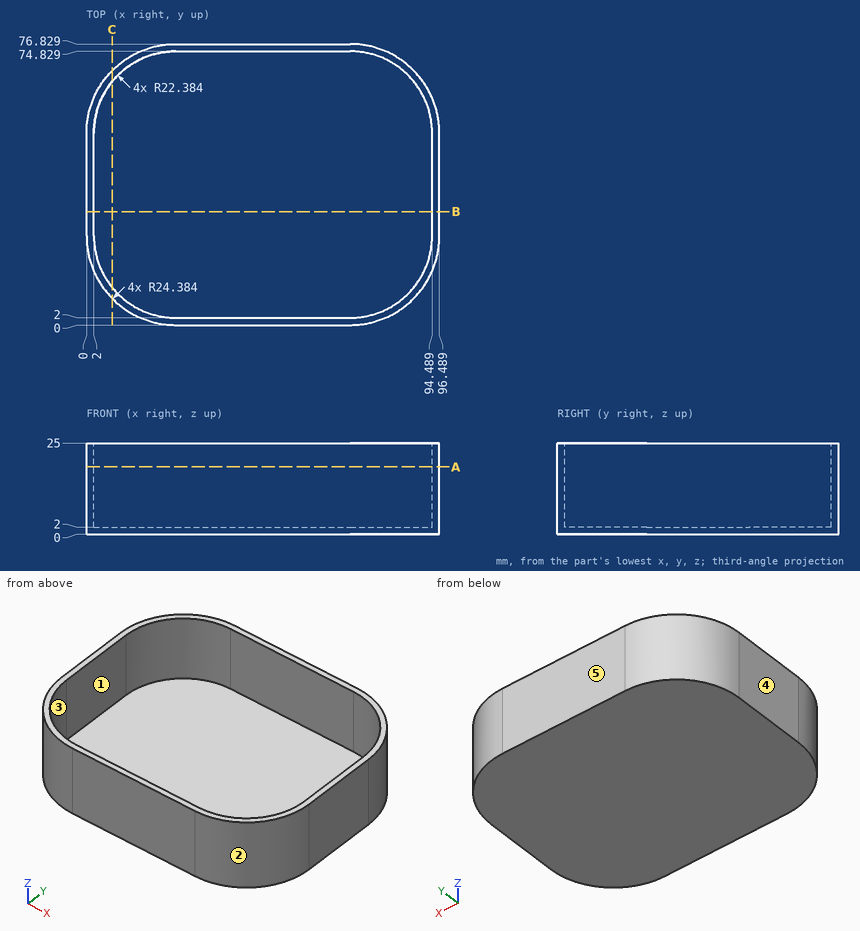
Print and shaded views of the part. All mm, measured from the part's lowest x, y and z. A direction names the side the tool comes from. Coordinates: 2 decimals unless noted, no trailing zeros. Loops run counter-clockwise (first coordinate to the right, second up) from the corner with the lowest first, then second, coordinate; pieces in that order, holes last. Notation, with made-up numbers: (59, 31.5) -> (112, 31.5) arc R35 ccw to (112, 70.5) -> close; hole circle Ø1 at (35, 60). An arc over 180 degrees is marked (long way). Use one line per item in the form item = value. Start each with the question number.
(1) Cut at A-A on z = 18.5. Give the cut face in (x, y) (1 decimal).
(2) Pull direction Y, two halves, no side cores. Call the marked faces 3, 4 and 5: pulls with the +Y half, pulls with the -Y half, needs draft (parallel to the pull), parting line crosses it, or undercut.
(3) Cut at B-B on y = 31. Give the cut face in (x, z), and give its area (3 significant figures).
(4) Cut at C-C on x = 7. Give the cut face in (y, z) (1 decimal).
(5) Tool access for the marked faces 1 and 2: list every direction of +Z, -Z, +X, -X, +Y, -Y with a clear straight run to the whole face (end or side of a thin tool).
(6) Flat gauge pins, fed straight in: pin 1 (8 mm diameter, centred on x = 85.5, z = 17.5, fed in from +Y); pin 2 (6 mm diameter, centred on y = 9, z = 5.5, fed in from -X); pin 3 (12 mm diameter, centred on x = 39, y = 30, fed in from +Z). Where does each tip first touch, or does it go through?
(7) Probe probe 1 along Y at (x, z) = (24, 21.5) (1 decimal); probe 2 along X at (y, z) = (45.5, 8); probe 3 along Z at (x, y) = (76, 57). List the from-to ranges inside material, lowest first. Write a range as from..to.
Values:
q1.outline = (0, 24.4) arc R24.4 ccw to (24.4, 0) -> (72.1, 0) arc R24.4 ccw to (96.5, 24.4) -> (96.5, 52.4) arc R24.4 ccw to (72.1, 76.8) -> (24.4, 76.8) arc R24.4 ccw to (0, 52.4) -> close; hole (2, 24.4) arc R22.4 ccw to (24.4, 2) -> (72.1, 2) arc R22.4 ccw to (94.5, 24.4) -> (94.5, 52.4) arc R22.4 ccw to (72.1, 74.8) -> (24.4, 74.8) arc R22.4 ccw to (2, 52.4) -> close
q2.face_3 = undercut
q2.face_4 = needs draft
q2.face_5 = pulls with the +Y half
q3.outline = (0, 0) -> (96.49, 0) -> (96.49, 25) -> (94.49, 25) -> (94.49, 2) -> (2, 2) -> (2, 25) -> (0, 25) -> close
q3.area = 285 mm2
q4.outline = (7.3, 0) -> (69.5, 0) -> (69.5, 25) -> (66.5, 25) -> (66.5, 2) -> (10.3, 2) -> (10.3, 25) -> (7.3, 25) -> close
q5.face_1 = +Z
q5.face_2 = +Z, -Z, +X, -Y
q6.pin_1 = 74.95
q6.pin_2 = 3.38
q6.pin_3 = 2
q7.probe_1 = 0..2, 74.8..76.8
q7.probe_2 = 0..2, 94.49..96.49
q7.probe_3 = 0..2
